Read the model definition and answer for the solid it produces. Units are mm, in the model's axes. Face numbers are marked on the shaded views. A direction names the side the tool comes from. Round coordinates to 2 decimals unless told otherwise and drop trailing zeros. Write each loop counter-clockwise with the first axis right and the second up, starting at its lowest first coordinate (ties: lowest second). Pieces come first, ordered by that corner, then holes. Notation, with made-up numbers: (82.25, 80.5) -> (132.25, 80.5) arc R14 cw to (132.25, 96.5) -> close; hole circle Ø8 at (-36, -23). An arc over 180 degrees is marked (long way). Return JSON: item names as keys, results as strings.
from build123d import *

# Parameters (mm, degrees)
SKETCH1_R           = 4
BOSS_EXTRUDE1_DEPTH = 12
BOSS_EXTRUDE3_DEPTH = 3


with BuildPart() as part:
    # Sketch1 → Boss-Extrude1 (new body)
    with BuildSketch(Plane(origin=(0, 0, 0), x_dir=(1, 0, 0), z_dir=(0, 1, 0))):
        with Locations(Location((0, 0, 0), (0, 0, 270))):
            Circle(SKETCH1_R)
    extrude(amount=BOSS_EXTRUDE1_DEPTH)

    # Sketch2 → Revolve1 (revolve)
    with BuildSketch(Plane.XY):
        with BuildLine():
            Line((0, 25.84428877), (0, 10.84428877))
            ThreePointArc((0, 10.84428877), (7.5, 18.34428877), (0, 25.84428877))
        make_face()
    revolve(axis=Axis((0, 25.84428877, 0), (0, -1, 0)))

    # Sketch4 → Boss-Extrude3 (add)
    with BuildSketch(Plane(origin=(0, 13, 0), x_dir=(-1, 0, 0), z_dir=(0, -1, 0))):
        Polygon((2.309401077, 4), (-2.309401077, 4), (-4.618802154, 0), (-2.309401077, -4), (2.309401077, -4), (4.618802154, 0), align=None)
    extrude(amount=BOSS_EXTRUDE3_DEPTH)


solid = part.part
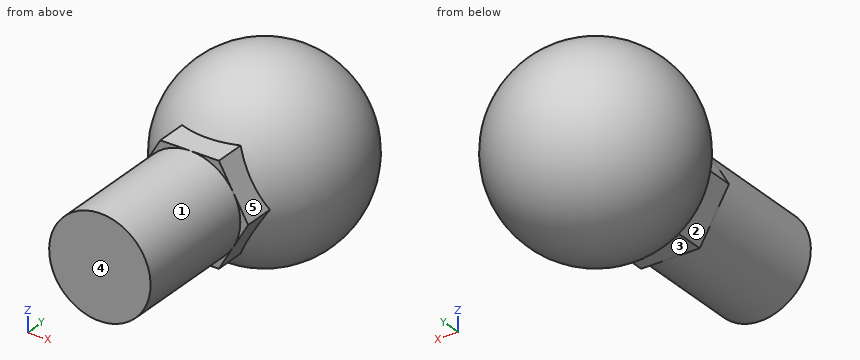
Item 1: Straight lines are drawn through the part: L1, parallel to Z at x = 0.5, y = 11.75; L2, parallel to Z at x = 2, y = 4.75; L3, parallel to Y at x = 2.25, z = 0.25. For each, find the intervals that lie inside material, in ascending order. Write a range as [from, to].
Worked answers:
{"L1": "z = [-4, 4]", "L2": "z = [-3.46, 3.46]", "L3": "y = [0, 25.49]"}
Item 2: For a pull along Z with two mould halves and no side action, classify the marked faces 3, 4 and 5 as released by +Z, released by -Z, zero draft, split by the parting line, or undercut.
Worked answers:
{"face 3": "released by -Z", "face 4": "zero draft", "face 5": "released by +Z"}
Item 3: Section A-A (z = 2.5) is taken. Give the vertices of the cut face in (x, y), then the cut area to 3 significant figures.
Worked answers:
{"outline": "(-3.18, 10) -> (-3.12, 10) -> (-3.12, 0) -> (3.12, 0) -> (3.12, 10) -> (3.18, 10) -> (3.18, 12.03) arc R7.07 ccw (long way) to (-3.18, 12.03) -> close", "area": "229 mm2"}
Item 4: Section D-D (x = -5.25) is taken. Give the vertices of the cut face in (y, z), then the cut area to 3 significant figures.
Worked answers:
{"outline": "circle Ø10.71 at (18.34, 0)", "area": "90.1 mm2"}
Item 5: A tool of negligible diameter and unlimited length cuts with its end or side. For the marked faces 1 and 2, from which of +Z, -Z, +X, -X, +Y, -Y can it reach the whole face along a straight path? Write none if from no direction.
Worked answers:
{"face 1": "-Y", "face 2": "-Z, -X, -Y"}
Item 6: Section B-B (y = 3.75) is taken. Give the vertices of the cut face in (x, z).
Worked answers:
{"outline": "circle Ø8 at (0, 0)"}
Item 7: Flat-ended cylindrical pins translate along their axes: pin 1 (1 mm diameter, centred on x = -1, y = 20.5, fed in from +Z); pin 2 (4 mm diameter, centred on x = -5, y = 16, fed in from -Z); pin 3 (5 mm diameter, centred on y = 10, z = -5, fed in from +X). Find the tip coordinate at first contact, or state that the pin passes through.
Worked answers:
{"pin 1": "stops at z = 7.26", "pin 2": "stops at z = -6.62", "pin 3": "stops at x = 3.18"}
